from build123d import *

# Parameters (mm, degrees)
F1_DEPTH  = 32.8
F2_R      = 22
F3_DEPTH  = 7.7
F4_R      = 19
F5_DEPTH  = 14
F7_DEPTH  = 29.8
F8_R      = 18
F9_DEPTH  = 7.7
F10_R     = 28
F11_DEPTH = 7
F12_R     = 2.1
F13_DEPTH = 39.801
F14_DEPTH = 11.1


with BuildPart() as f1:
    # F0 (on Top) → F1 (new body)
    with BuildSketch(Plane.XY):
        with BuildLine():
            Line((-43, -20), (-18.1383571472, -20))
            ThreePointArc((-18.1383571472, -20), (27, 0), (-18.1383571472, 20))
            Line((-18.1383571472, 20), (-43, 20))
            ThreePointArc((-43, 20), (-63, 0), (-43, -20))
        make_face()
    extrude(amount=F1_DEPTH)

    # F2 (on face) → F3 (cut)
    with BuildSketch(Plane.XY.offset(32.8)):
        Circle(F2_R)
    extrude(amount=-F3_DEPTH, mode=Mode.SUBTRACT)

    # F4 (on face) → F5 (cut)
    with BuildSketch(Plane.XY.offset(25.1)):
        Circle(F4_R)
    extrude(amount=-F5_DEPTH, mode=Mode.SUBTRACT)

    # F6 (on face) → F7 (cut)
    with BuildSketch(Plane.XY.offset(32.8)):
        with BuildLine():
            Line((-60, -7.3), (-54.9461290802, -7.3))
            ThreePointArc((-54.9461290802, -7.3), (-29, 0), (-54.9461290802, 7.3))
            Line((-54.9461290802, 7.3), (-60, 7.3))
            Line((-60, 7.3), (-60, -7.3))
        make_face()
    extrude(amount=-F7_DEPTH, mode=Mode.SUBTRACT)

    # F8 (on face) → F9 (cut)
    with BuildSketch(Plane.XY.offset(32.8)):
        with Locations((-35, 0)):
            Circle(F8_R)
    extrude(amount=-F9_DEPTH, mode=Mode.SUBTRACT)

    # F10 (on face) → F11 (join)
    with BuildSketch(Plane(origin=(0, 0, 0), x_dir=(1, 0, 0), z_dir=(0, 0, -1))):
        Circle(F10_R)
        with BuildLine():
            ThreePointArc((0.8760965756, 5.5), (17, 0), (0.8760965756, -5.5))
            Line((0.8760965756, -5.5), (-11.4999995261, -5.5))
            ThreePointArc((-11.4999995261, -5.5), (-17, 0), (-11.4999995261, 5.5))
            Line((-11.4999995261, 5.5), (0.8760965756, 5.5))
        make_face(mode=Mode.SUBTRACT)
    extrude(amount=F11_DEPTH)

    # F12 (on face) → F13 (cut, through all)
    with BuildSketch(Plane(origin=(0, 0, -7), x_dir=(1, 0, 0), z_dir=(0, 0, -1))):
        with Locations((0, -19.5)):
            Circle(F12_R)
        with Locations((0, 19.5)):
            Circle(F12_R)
    extrude(amount=-F13_DEPTH, mode=Mode.SUBTRACT)

    # F14 (cut, through all): a face of the model
    f14_faces = [f1.faces().sort_by_distance(p)[0] for p in [
        (1.5412658512, 0, 0),
    ]]
    extrude(f14_faces, amount=-F14_DEPTH, mode=Mode.SUBTRACT)


solid = f1.part
The model under review builds one solid part; all positions refer to its coordinate system, in mm. A direction names the side the tool comes from. Coordinates: 2 decimals unless noted, no trailing zeros. Order: outer loops, then holes, each group sorted by start corner. A loop starts at its lowest first (then second) coordinate and runs counter-clockwise, first axis right, second up. Notation, with made-up numbers: (66, 61.25) -> (75, 61.25) arc R12 cw to (75, 82.25) -> close; hole circle Ø7 at (19, -1). An arc over 180 degrees is marked (long way). Answer in a Markdown table with one row per item.
(1) Wall thickness on line 1 along Y through (x, z) = (0, 7.5); line 2 along Y through (x, z) = (0, 31.25); line 3 along X through (y, z) = (12, 23): over which ranges is each line inside the solid? List them lowest first.
Answers:
| item | result |
|---|---|
| line 1 | -27 to -21.6, -17.4 to -5.5, 5.5 to 17.4, 21.6 to 27 |
| line 2 | -27 to -22, 22 to 27 |
| line 3 | -59 to -50.21, -35.79 to -14.73, 14.73 to 24.19 |
(2) Consider section A-A (z = 19). Write out the cut boundary in (x, y), plus the area to 3 significant figures.
Answers:
| item | result |
|---|---|
| outline | (-43, -20) -> (-18.14, -20) arc R27 ccw (long way) to (-18.14, 20) -> (-43, 20) arc R20 ccw to start; hole (-60, -7.3) -> (-54.95, -7.3) arc R14 ccw (long way) to (-54.95, 7.3) -> (-60, 7.3) -> close; hole (-2.01, -18.89) arc R2.1 ccw (long way) to (2.01, -18.89) arc R19 ccw to (2.01, 18.89) arc R2.1 ccw (long way) to (-2.01, 18.89) arc R19 ccw to start |
| area | 1,850 mm² |
(3) The part is to be moulded in two halves that separate along X. For faces 4 (the cylindrical face through (-19, 0, 18)), 5 (the flat face through (0, 6, -7)), 6 (the cylindrical face through (-63, 0, 16)), say which applies: +X half, -X half, draft (parallel to the pull), parting line (faces both ways), or undercut.
Answers:
| item | result |
|---|---|
| face 4 | undercut |
| face 5 | draft |
| face 6 | -X half |
(4) Consider section C-C (x = 8). Write out the cut boundary in (y, z).
Answers:
| item | result |
|---|---|
| outline | (-26.83, -7) -> (-9, -7) -> (-9, 11.1) -> (-17.23, 11.1) -> (-17.23, 25.1) -> (-20.49, 25.1) -> (-20.49, 32.8) -> (-25.79, 32.8) -> (-25.79, 0) -> (-26.83, 0) -> close; (9, -7) -> (26.83, -7) -> (26.83, 0) -> (25.79, 0) -> (25.79, 32.8) -> (20.49, 32.8) -> (20.49, 25.1) -> (17.23, 25.1) -> (17.23, 11.1) -> (9, 11.1) -> close |
(5) Machinability: for faces 1 (the flat face through (-22, -14, 32.8)), 2 (the flat face through (-57, 7.3, 18)), 3 (the flat face through (-5, 5.5, 2)), which of the approach directions +Z, -Z, +X, -X, +Y, -Y give a long, thin tool a straight path to every point of the face, cutting with its end or side? Answer none if there is none.
Answers:
| item | result |
|---|---|
| face 1 | +Z, +X, -X, +Y, -Y |
| face 2 | +Z |
| face 3 | +Z, -Z |
(6) Consider section D-D (z = 28). Write out the cut boundary in (x, y), plus the area to 3 significant figures.
Answers:
| item | result |
|---|---|
| outline | (-43, -20) -> (-18.14, -20) arc R27 ccw (long way) to (-18.14, 20) -> (-43, 20) arc R20 ccw to start; hole (-60, -7.3) -> (-54.95, -7.3) arc R14 ccw to (-47, -13.42) arc R18 ccw to (-19.79, -9.62) arc R22 ccw (long way) to (-19.79, 9.62) arc R18 ccw to (-47, 13.42) arc R14 ccw to (-54.95, 7.3) -> (-60, 7.3) -> close |
| area | 1,050 mm² |
(7) Consider section B-B (z = 10). Write out the cut boundary in (x, y), plus the area to 3 significant figures.
Answers:
| item | result |
|---|---|
| outline | (-43, -20) -> (-18.14, -20) arc R27 ccw (long way) to (-18.14, 20) -> (-43, 20) arc R20 ccw to start; hole (-60, -7.3) -> (-54.95, -7.3) arc R14 ccw (long way) to (-54.95, 7.3) -> (-60, 7.3) -> close; hole (-11.5, -5.5) -> (0.88, -5.5) arc R9 ccw (long way) to (0.88, 5.5) -> (-11.5, 5.5) arc R5.5 ccw to start; hole circle Ø4.2 at (0, -19.5); hole circle Ø4.2 at (0, 19.5) |
| area | 2,550 mm² |
(8) Insertion check: pin 1 (20 mm diameter, centred on x = -35, z = 22.5, fed in from +Y); pin 2 (16 mm diameter, centred on y = 3.5, z = 16, fed in from +X); pin 3 (22 mm diameter, centred on x = -3.5, y = 8.5, fed in from +Z); pin 4 (16 mm diameter, centred on x = 8, y = 0, fed in from -Z). Each pin has a flat end and moves straight along its axis. Give the tip position at first contact, or say it passes through.
Answers:
| item | result |
|---|---|
| pin 1 | y = 20 |
| pin 2 | x = 27 |
| pin 3 | z = 25.1 |
| pin 4 | through |
